Input: part model. Units: mm. Frame: model coordinates. A direction names the side the tool comes from. Give positions to 0.01 mm unless a question says otherwise; leave off trailing zeros. Loops run counter-clockwise (first coordinate to the right, second up) from the corner with the lowest first, then second, coordinate; pieces in that order, holes last. Notation, with made-up numbers: (-29.5, -34) - (21.5, -34) arc R16 cw to (21.5, -28) - close; hole circle Ø8 at (1, -34.75). An arc over 180 degrees is marked (long way). One line per question, with ' | ' between items. Start each with the question number.
from build123d import *

# Parameters (mm, degrees)
F0_W     = 1524
F0_H     = 914.4
F1_DEPTH = 50.8
F2_W     = 50.8
F2_H     = 50.8
F3_DEPTH = 698.5


with BuildPart() as f1:
    # F0 (on Top) → F1 (new body)
    with BuildSketch(Plane.XY):
        with Locations((27.529123, 0.555292)):
            Rectangle(F0_W, F0_H)
    extrude(amount=F1_DEPTH)

    # F2 (on face) → F3 (join)
    with BuildSketch(Plane.XY.offset(50.8)):
        with Locations((-658.270877, -380.444708)):
            Rectangle(F2_W, F2_H)
    extrude(amount=-F3_DEPTH)

    # F4: F1 across plane


with BuildPart() as f1_1:
    add(f1.part)
    add(f1.part.mirror(Plane.XZ))

    # F5: F1 across plane


with BuildPart() as f1_2:
    add(f1_1.part)
    add(f1_1.part.mirror(Plane.YZ))


solid = f1_2.part
Q1. Line query: L1, parallel to Y at x = 637.5, z = -307; L2, parallel to Z at x = 465, y = -115. Output: solid intervals per line, ascending. Write a range as from..to.
Q2. Draft query along X for faces 1 (the face through (-659, 405.845, -319)), 2 (the face through (683.671, -381, -319)), 3 (the face through (632.871, -381, -319)). Return one class per face: +X half, -X half, draft (parallel to the pull), parting line (faces both ways), or undercut.
Q3. Section B-B, the plane y = 103.5. Output: boundary loops of the cut face in (x, z).
Q4. First-contact query: pin 1 (3 mm diameter, centred on x = -524, y = -66.5, fed in from -Z); pin 2 (15 mm diameter, centred on x = -651, z = -402.5, fed in from +Y). Flat tips, straight axial feed; report the tip coordinate or a pass-through.
Q5. Section C-C, the plane x = 14. Output: boundary loops of the cut face in (y, z).
Q6. Section A-A, the plane z = -219.5. Output: boundary loops of the cut face in (x, y).
Q7. Access query for faces 4 (the face through (659, -405.845, -319)), 5 (the face through (659, -355.045, -319)), 6 (the face through (683.671, 381, -319)), 7 (the face through (-632.871, -381, -319)), 8 (the face through (-683.671, -381, -319)). Directions: +Z, -Z, +X, -X, +Y, -Y. A direction counts if a zero-diameter tool reaches every point of the face in a straight line with its end or side. Return the directions, or none.
Solved:
1) L1: y = -405.84..-355.04, 355.04..405.84 | L2: z = 0..50.8
2) face 1: draft | face 2: +X half | face 3: undercut
3) outline: (-789.53, 0) - (789.53, 0) - (789.53, 50.8) - (-789.53, 50.8) - close
4) pin 1: stops at z = 0 | pin 2: stops at y = 405.84
5) outline: (-457.76, 0) - (457.76, 0) - (457.76, 50.8) - (-457.76, 50.8) - close
6) outline: (-683.67, -405.84) - (-632.87, -405.84) - (-632.87, -355.04) - (-683.67, -355.04) - close; (-683.67, 355.04) - (-632.87, 355.04) - (-632.87, 405.84) - (-683.67, 405.84) - close; (632.87, -405.84) - (683.67, -405.84) - (683.67, -355.04) - (632.87, -355.04) - close; (632.87, 355.04) - (683.67, 355.04) - (683.67, 405.84) - (632.87, 405.84) - close
7) face 4: -Z, +X, -X, -Y | face 5: -Z, +X, -X | face 6: -Z, +X, +Y, -Y | face 7: -Z, +Y, -Y | face 8: -Z, -X, +Y, -Y
